```python
from build123d import *

# Parameters (mm, degrees)
F1_DEPTH = 304.8
F3_D     = 7.62
F3_DEPTH = 25.4


with BuildPart() as f1:
    # F0 (on Top) → F1 (new body)
    with BuildSketch(Plane.XY):
        with BuildLine():
            Line((-4.8895, -9.525), (4.8895, -9.525))
            Line((4.8895, -9.525), (4.8895, -6.861627))
            ThreePointArc((4.8895, -6.861627), (4.593677, -6.366351), (4.8895, -5.871076))
            Line((4.8895, -5.871076), (4.8895, 5.871076))
            ThreePointArc((4.8895, 5.871076), (4.593677, 6.366351), (4.8895, 6.861627))
            Line((4.8895, 6.861627), (4.8895, 9.525))
            Line((4.8895, 9.525), (-4.8895, 9.525))
            Line((-4.8895, 9.525), (-4.8895, 4.445))
            Line((-4.8895, 4.445), (-2.54, 4.445))
            Line((-2.54, 4.445), (-2.54, 6.35))
            Line((-2.54, 6.35), (2.54, 6.35))
            Line((2.54, 6.35), (2.54, -6.35))
            Line((2.54, -6.35), (-2.54, -6.35))
            Line((-2.54, -6.35), (-2.54, -4.445))
            Line((-2.54, -4.445), (-4.8895, -4.445))
            Line((-4.8895, -4.445), (-4.8895, -9.525))
        make_face()
    extrude(amount=F1_DEPTH)

    # F3
    with Locations(Plane.YZ.offset(4.8895)):
        with Locations((0, 295.275), (0, 142.875), (0, 73.025), (0, 9.525)):
            Hole(F3_D / 2, depth=F3_DEPTH)


solid = f1.part
```
Can you work these out from the model? Positions are in its coordinate system, mm. A direction names the side the tool comes from. Coordinates: 2 decimals unless noted, no trailing zeros. Loops run counter-clockwise (first coordinate to the right, second up) from the corner with the lowest first, then second, coordinate; pieces in that order, holes last. Notation, with made-up numbers: (65.25, -19) - (91.25, -19) arc R17 ccw to (91.25, 5) - close; hole circle Ø11 at (56, 14.5). An arc over 180 degrees is marked (long way). Use a Markdown table: item, result.
Item 1: For faces 1 (the face through (3.698, 0.496, 146.653)), 2 (the face through (0, 6.35, 150)), which set-ups out of +Z, -Z, +X, -X, +Y, -Y let a thin tool reach every point of the face, with its end or its side?
Numbers:
| item | result |
|---|---|
| face 1 | +X, -X |
| face 2 | +Z, -Z |
Item 2: Will this pin go through, and if not, where does the flat tip stop? pin 1 (4.5 mm diameter, centred on y = 0, z = 142.875, fed in from +X).
Numbers:
| item | result |
|---|---|
| pin 1 | passes through |
Item 3: We'd pull the mould along Y, two halves only. Please class faces 3 (the face through (0, -6.35, 150)), 4 (the face through (0, -9.525, 150)), 5 (the face through (3, 0, 304.8)), 6 (the face through (2.54, 0, 150)): released by +Y, released by -Y, zero draft, split by the parting line, or undercut.
Numbers:
| item | result |
|---|---|
| face 3 | undercut |
| face 4 | released by -Y |
| face 5 | zero draft |
| face 6 | undercut |
Item 4: I want a section at A-A on y = 0. Please give me the cut outline in (x, z) (1 decimal).
Numbers:
| item | result |
|---|---|
| outline | (2.5, 0) - (4.9, 0) - (4.9, 5.7) - (2.5, 5.7) - close; (2.5, 13.3) - (4.9, 13.3) - (4.9, 69.2) - (2.5, 69.2) - close; (2.5, 76.8) - (4.9, 76.8) - (4.9, 139.1) - (2.5, 139.1) - close; (2.5, 146.7) - (4.9, 146.7) - (4.9, 291.5) - (2.5, 291.5) - close; (2.5, 299.1) - (4.9, 299.1) - (4.9, 304.8) - (2.5, 304.8) - close |
Item 5: I want a section at B-B on x = 0.5. Please give me the cut outline in (y, z) (3 decimals).
Numbers:
| item | result |
|---|---|
| outline | (-9.525, 0) - (-6.35, 0) - (-6.35, 304.8) - (-9.525, 304.8) - close; (6.35, 0) - (9.525, 0) - (9.525, 304.8) - (6.35, 304.8) - close |
Item 6: If I drill on probe 1 along Z at (x, y) = (4, 0) (3 decimals); probe 2 along Y at (x, z) = (1.5, 176) (3 decimals); probe 3 along X at (y, z) = (-5.25, 108.5), over which ranges is the centre line in solid material (lowest first)? Write a range as from..to.
Numbers:
| item | result |
|---|---|
| probe 1 | z = 0..5.715, 13.335..69.215, 76.835..139.065, 146.685..291.465, 299.085..304.8 |
| probe 2 | y = -9.525..-6.35, 6.35..9.525 |
| probe 3 | x = -4.89..-2.54, 2.54..4.89 |
